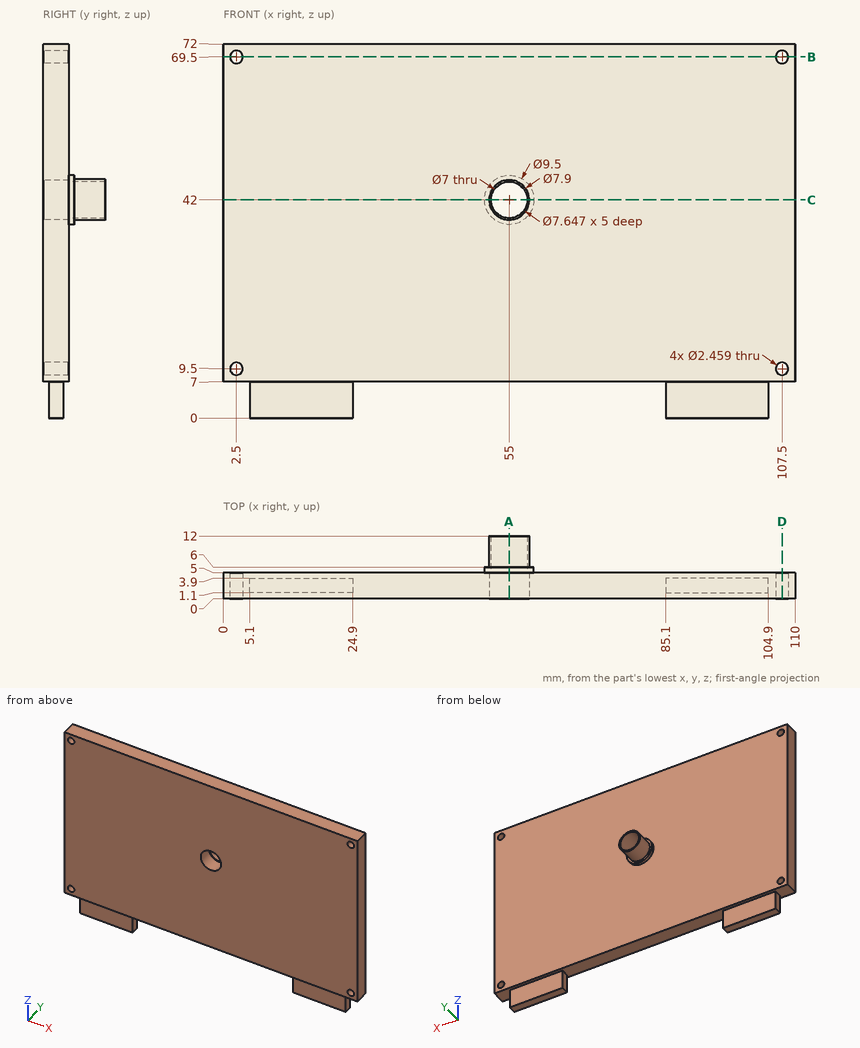
Here's the drawing with two shaded views (mm, measured from the low corner). I have some questions. Give positions to 0.01 mm unless a question says otherwise; leave off trailing zeros. Write each loop counter-clockwise with the first axis right and the second up, starting at its lowest first coordinate (ties: lowest second). Pieces come first, ordered by that corner, then holes. Notation, with made-up numbers: (36.5, 46) -> (50.5, 46) arc R14 cw to (50.5, 65) -> close; hole circle Ø2 at (-35.75, 85). An arc over 180 degrees is marked (long way). Answer as a JSON object with one key per item and string values. Group by question number.
Item 1: Suppose I cut it at B-B (z = 69.5). Please give me the cut outline in (x, y).
Item 2: Suppose I cut it at C-C (z = 42). Please give me the cut outline in (x, y), plus the area to 3 significant figures.
Item 3: Suppose I cut it at D-D (x = 107.5). Please give me the cut outline in (y, z), plus the area to 3 significant figures.
Item 4: I'm going to push flat-ended pins straight in: P1, Ø1.4, axis at y = 2.5, z = 3.5, coming from the -X side; P2, Ø2, axis at x = 93, z = 5, coming from the -Y side; P3, Ø3.5, axis at x = 99.5, z = 3, coming from the +Y side. Where does each tip first touch, or does it pass through?
Item 5: Please list where these lines run through material, in increasing order: line 1 (Z direction, x = 107.5, y = 3.35); line 2 (X direction, y = 3.1, z = 69.5); line 3 (X direction, y = 3.25, z = 42). Write a range as [from, to].
Item 6: Suppose I cut it at A-A (x = 55). Please give me the cut outline in (y, z).
Findings:
{
 "1": {"outline": "(0, 0) -> (1.27, 0) -> (1.27, 5) -> (0, 5) -> close; (3.73, 0) -> (106.27, 0) -> (106.27, 5) -> (3.73, 5) -> close; (108.73, 0) -> (110, 0) -> (110, 5) -> (108.73, 5) -> close"},
 "2": {"outline": "(0, 0) -> (51.18, 0) -> (51.18, 5) -> (51.5, 5) -> (51.5, 12) -> (51.05, 12) -> (51.05, 6) -> (50.25, 6) -> (50.25, 5) -> (0, 5) -> close; (58.5, 5) -> (58.82, 5) -> (58.82, 0) -> (110, 0) -> (110, 5) -> (59.75, 5) -> (59.75, 6) -> (58.95, 6) -> (58.95, 12) -> (58.5, 12) -> close", "area": "520 mm²"},
 "3": {"outline": "(0, 7) -> (5, 7) -> (5, 8.27) -> (0, 8.27) -> close; (0, 10.73) -> (5, 10.73) -> (5, 68.27) -> (0, 68.27) -> close; (0, 70.73) -> (5, 70.73) -> (5, 72) -> (0, 72) -> close", "area": "300 mm²"},
 "4": {"P1": "stops at x = 5.1", "P2": "stops at y = 1.1", "P3": "stops at y = 3.9"},
 "5": {"line 1": "z = [7, 8.27], [10.73, 68.27], [70.73, 72]", "line 2": "x = [0, 1.27], [3.73, 106.27], [108.73, 110]", "line 3": "x = [0, 51.18], [58.82, 110]"},
 "6": {"outline": "(0, 7) -> (5, 7) -> (5, 37.25) -> (6, 37.25) -> (6, 38.05) -> (12, 38.05) -> (12, 38.5) -> (5, 38.5) -> (5, 38.18) -> (0, 38.18) -> close; (0, 45.82) -> (5, 45.82) -> (5, 45.5) -> (12, 45.5) -> (12, 45.95) -> (6, 45.95) -> (6, 46.75) -> (5, 46.75) -> (5, 72) -> (0, 72) -> close"}
}
